The model under review builds one solid part; all positions refer to its coordinate system, in mm. Face numbers are marked on the shaded views. A direction names the side the tool comes from. Give positions to 0.01 mm unless a question says otherwise; leave off trailing zeros. Order: outer loops, then holes, each group sorted by start corner. A loop starts at its lowest first (then second) coordinate and runs counter-clockwise, first axis right, second up.
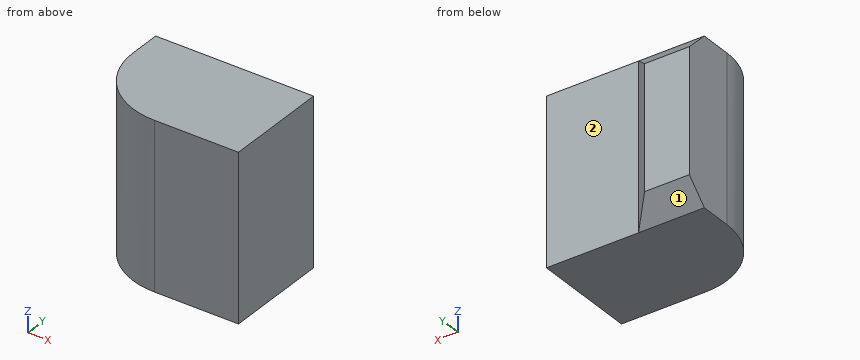
```python
from build123d import *

# Parameters (mm, degrees)
BOSS_EXTRUDE1_DEPTH      = 117
BOSS_EXTRUDE1_DEPTH_BACK = 117
SKETCH1_W                = 350
SKETCH1_H                = 300
BOSS_EXTRUDE2_DEPTH      = 200
BOSS_EXTRUDE2_DEPTH_BACK = 200
CUT_EXTRUDE1_DEPTH       = 540
CUT_EXTRUDE2_DEPTH       = 138
CUT_EXTRUDE2_DEPTH_BACK  = 540
CHAMFER1_SIZE            = 40
CHAMFER2_SIZE            = 40
FILLET1_R                = 140
CUT_EXTRUDE3_DEPTH       = 602.0000000000001
CUT_EXTRUDE4_DEPTH       = 602.0000000000001


with BuildPart() as part:
    # Sketch1 → Boss-Extrude1 (new, two sides: drawn at the far end of the back side and taken through both)
    with BuildSketch(Plane.XY.offset(-BOSS_EXTRUDE1_DEPTH_BACK)):
        Rectangle(SKETCH1_W, SKETCH1_H)
    extrude(amount=BOSS_EXTRUDE1_DEPTH + BOSS_EXTRUDE1_DEPTH_BACK)

    # Sketch3 → Boss-Extrude2 (add, two sides: drawn at the far end of the back side and taken through both)
    with BuildSketch(Plane(origin=(0, 0, 0), x_dir=(-1, 0, 0), z_dir=(0, 0, -1)).offset(-BOSS_EXTRUDE2_DEPTH_BACK)):
        Polygon((-175, 150), (-175, -150), (175, -150), (174.99999999999997, 50.00000000000006), (-75.00000000000003, 50.000000000000014), (-75.00000000000004, 150), align=None)
    extrude(amount=BOSS_EXTRUDE2_DEPTH + BOSS_EXTRUDE2_DEPTH_BACK)

    # Sketch4 → Cut-Extrude1 (cut)
    with BuildSketch(Plane(origin=(0, 0, -117), x_dir=(-1, 0, 0), z_dir=(0, 0, -1))):
        Polygon((174.99999999999997, 150), (-75.00000000000004, 149.99999999999997), (-75.00000000000004, 89.99999999999997), (174.99999999999997, 90), align=None)
    extrude(amount=-CUT_EXTRUDE1_DEPTH, mode=Mode.SUBTRACT)

    # Sketch6 → Cut-Extrude2 (cut, two sides: drawn at the far end of the back side and taken through both)
    with BuildSketch(Plane(origin=(0, 0, -117), x_dir=(-1, 0, 0), z_dir=(0, 0, -1)).offset(-CUT_EXTRUDE2_DEPTH_BACK)):
        Polygon((-188.8193544446854, 158.10037053286104), (89.99999999999997, 158.10037053286104), (89.99999999999997, 50.00000000000004), (-188.8193544446854, 50.00000000000003), align=None)
    extrude(amount=CUT_EXTRUDE2_DEPTH + CUT_EXTRUDE2_DEPTH_BACK, mode=Mode.SUBTRACT)

    # Chamfer1
    chamfer1_edges = [part.edges().sort_by_distance(p)[0] for p in [
        (-89.99999999999997, 50.00000000000004, 0),
    ]]
    chamfer(chamfer1_edges, length=CHAMFER1_SIZE - 0.0001)  # a hair under: the kernel refuses the full size

    # Chamfer2
    chamfer2_edges = [part.edges().sort_by_distance(p)[0] for p in [
        (-112.50004999999997, 50.00000000000004, 117),
        (-112.50004999999997, 50.00000000000004, -117),
    ]]
    chamfer(chamfer2_edges, length=CHAMFER2_SIZE - 0.0001)  # a hair under: the kernel refuses the full size

    # Fillet1
    fillet1_edges = [part.edges().sort_by_distance(p)[0] for p in [
        (-175, -150, 0),
    ]]
    fillet(fillet1_edges, radius=FILLET1_R)

    # Sketch7 → Cut-Extrude3 (cut)
    with BuildSketch(Plane(origin=(0, 0, -200), x_dir=(-1, 0, 0), z_dir=(0, 0, -1))):
        Polygon((-124.99999999999997, 50.00000000000004), (-124.99999999999996, -150), (-196.63418814024195, -174.37612145790905), (-210.87565010922705, 102.36305485317497), align=None)
    extrude(amount=-CUT_EXTRUDE3_DEPTH, mode=Mode.SUBTRACT)

    # Sketch8 → Cut-Extrude4 (cut)
    with BuildSketch(Plane.ZY.offset(174.99999999999997)):
        Polygon((156.99999999999991, 50.00000000000004), (156.99999999999991, -180.65334412999255), (404.27559038441177, -197.1355795745069), (273.0172818180443, 154.636687383358), align=None)
        Polygon((-157.00000000000037, 50.00000000000004), (-157.00000000000037, -188.89446185224972), (-332.7435139552091, -205.02559262419945), (-278.28880023445754, 167.10797834540983), align=None)
    extrude(amount=-CUT_EXTRUDE4_DEPTH, mode=Mode.SUBTRACT)


solid = part.part
```
Item 1: Take a section at D-D (x = 98.5). Give the boundary of the cut face in (y, z).
Values found:
outline: (-150, -157) - (50, -157) - (50, 157) - (-150, 157) - close
Item 2: Take a section at C-C (y = -51). Give the boundary of the cut face in (x, z), and give its area (3 significant figures).
Values found:
outline: (-168.86, -157) - (125, -157) - (125, 157) - (-168.86, 157) - close
area: 92,300 mm2
Item 3: For line 1 (Y direction, x = -0.5, z = 66); line 2 (X direction, y = 59, z = 89); line 3 (Y direction, x = -81, z = 68.5), list the stretches that pass through material, from the lowest coordinate up.
Values found:
line 1: y = -150 to 50
line 2: x = -175 to -59
line 3: y = -142.23 to 81
Item 4: For the marked faces 1 and 2, list the 3-axis set-ups (+Z, -Z, +X, -X, +Y, -Y) from which the entire face can be reached by the end or side of a thin tool; tool diameter is ignored.
Values found:
face 1: -Z, +X, -X, +Y
face 2: +Z, -Z, +X, +Y
Item 5: Clearance check with flat-ended pins moving along their axes: pin 1 Ø1 at (x, z) = (-67.5, -105.5) entering from +Y; pin 2 Ø2 at (x, z) = (50.5, -73.5) entering from +Y. State where each tip first meets the part, or that it passes through.
Values found:
pin 1: stops at y = 68
pin 2: stops at y = 50
